Autodesk Fusion 360 part; units mm, degrees
sketch "Sketch1" plane through (0, 0, 0) normal (0, 0, 1) x (1, 0, 0)
  line L0 (0, 0) -> (0, -100)
  line L1 (0, -100) -> (-50, -100)
  line L2 (-100, -100) -> (-150, -100)
  line L3 (-150, -100) -> (-150, -50)
  line L4 (-150, -50) -> (-190, -30)
  line L5 (-190, -30) -> (-190, 0)
  line L6 (-190, 0) -> (0, 0)
  line L7 (-50, -100) -> (-50, -70)
  line L8 (-50, -70) -> (-100, -70)
  line L9 (-100, -70) -> (-100, -100)
revolve "Revolve1" add sketch "Sketch1" angle 360 about axis through (-190, 0, 0) along (1, 0, 0)
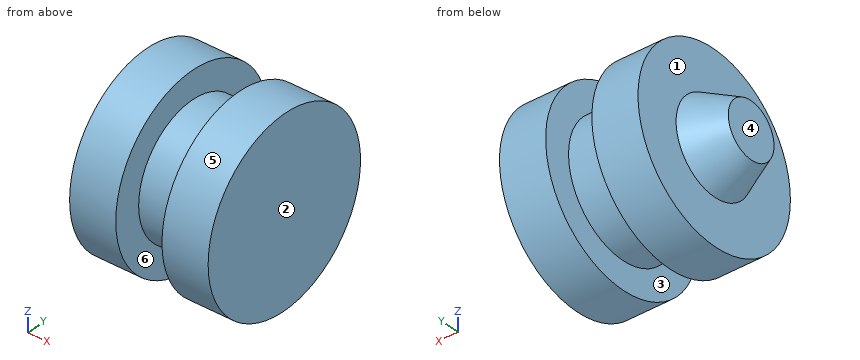
The listing builds one solid part. Answer for the finished solid, in the listing's coordinates (mm). Face numbers are marked on the shaded views. A direction names the side the tool comes from. Coordinates: 2 decimals unless noted, no trailing zeros. Loops run counter-clockwise (first coordinate to the right, second up) from the corner with the lowest first, then second, coordinate; pieces in that order, holes last. Notation, with made-up numbers: (66.5, -12) -> (75.5, -12) arc R12 cw to (75.5, -4) -> close; hole circle Ø5 at (-4.5, 51.5). An arc over 180 degrees is marked (long way). Answer in a Markdown table with one row per item. Add a question column.
1. For the marked faces 1, 2 and 3, determine the directions among +Z, -Z, +X, -X, +Y, -Y from which every point of the face is accessible in a straight line to the end or side of a thin tool.
2. The part is cut by section A-A, the plane y = 0. Write down the section's boundary in (x, z), then the cut area to 3 significant figures.
3. Consider line 1 (X direction, y = 26, z = 79); line 2 (Z direction, x = -35, y = -1) (3 decimals); line 3 (X direction, y = 0, z = -30). Determine where each line is inside the solid, lowest interval first. Write a range as [from, to].
4. The part is cut by section C-C, the plane z = 86. Write down the section's boundary in (x, y), then the cut area to 3 significant figures.
5. Determine the mould class of the marked faces 4, 5 and 6 for opening direction X: +X half, -X half, draft (parallel to the pull), parting line (faces both ways), or undercut.
6. Flat-ended cylindrical pins translate along their axes: P1, Ø4, axis at y = -16.5, z = 30, coming from the -X side; P2, Ø3, axis at x = -94, z = -19.5, coming from the -Y side; P3, Ø1, axis at x = -145, z = 3.5, coming from the -Y side (3 decimals). Find the tip coordinate at first contact, or state that the pin passes through.
7. The part is cut by section D-D, the plane x = -111. Write down the section's boundary in (y, z).
Answer below:
| question | item | result |
|---|---|---|
| 1 | face 1 | -X |
| 1 | face 2 | +Z, -Z, +X, +Y, -Y |
| 1 | face 3 | none |
| 2 | outline | (-190, -30) -> (-150, -50) -> (-150, -100) -> (-100, -100) -> (-100, -70) -> (-50, -70) -> (-50, -100) -> (0, -100) -> (0, 100) -> (-50, 100) -> (-50, 70) -> (-100, 70) -> (-100, 100) -> (-150, 100) -> (-150, 50) -> (-190, 30) -> close |
| 2 | area | 30,200 mm2 |
| 3 | line 1 | [-150, -100], [-50, 0] |
| 3 | line 2 | [-99.995, 99.995] |
| 3 | line 3 | [-190, 0] |
| 4 | outline | (-150, -51.03) -> (-100, -51.03) -> (-100, 51.03) -> (-150, 51.03) -> close; (-50, -51.03) -> (0, -51.03) -> (0, 51.03) -> (-50, 51.03) -> close |
| 4 | area | 10,200 mm2 |
| 5 | face 4 | -X half |
| 5 | face 5 | draft |
| 5 | face 6 | undercut |
| 6 | P1 | x = -185.52 |
| 6 | P2 | y = -67.65 |
| 6 | P3 | y = -99.955 |
| 7 | outline | circle Ø200 at (0, 0) |
